Answer from the drawing. Dimensions are ordinates in mm from the lowest x, y and z of the part. A direction names the side the tool comes from. Round coordinates to 2 decimals unless told otherwise and drop trailing zeros. Write each loop counter-clockwise with the first axis right and the second up, starting at its lowest first coordinate (ties: lowest second). Pieces come first, ordered by that corner, then holes. Notation, with made-up numbers: (-9, 43.5) - (48, 43.5) arc R10 ccw to (48, 61.5) - close; hole circle Ø3 at (35, 13). An arc over 180 degrees is marked (long way). Answer in a Markdown table with one row per item.
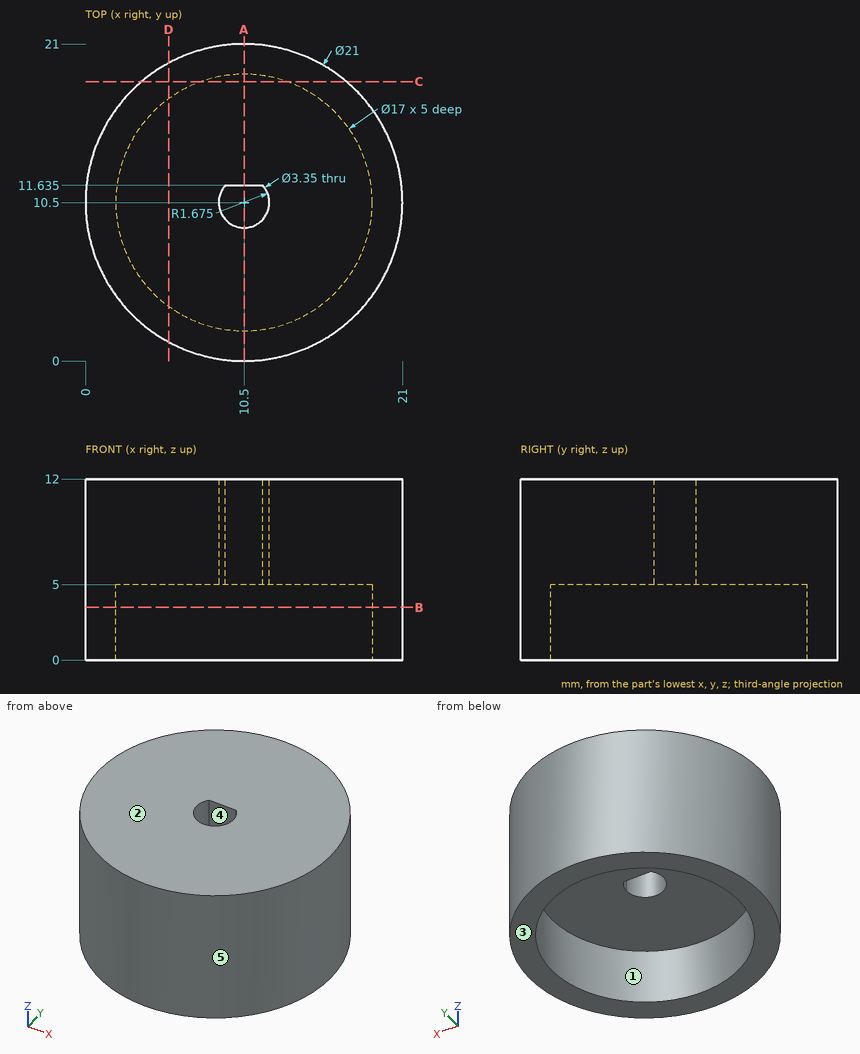
(1) Section B-B (z = 3.5) is taken. Give the vertices of the cut face in (x, y), and give its area (3 significant figures).
Checked values:
| item | result |
|---|---|
| outline | circle Ø21 at (10.5, 10.5); hole circle Ø17 at (10.5, 10.5) |
| area | 119 mm2 |
(2) Section A-A (x = 10.5) is taken. Give the vertices of the cut face in (y, z) (1 decimal), and give its area (3 significant figures).
Checked values:
| item | result |
|---|---|
| outline | (0, 0) - (2, 0) - (2, 5) - (8.8, 5) - (8.8, 12) - (0, 12) - close; (11.6, 5) - (19, 5) - (19, 0) - (21, 0) - (21, 12) - (11.6, 12) - close |
| area | 147 mm2 |
(3) For a pull along X with two mould halves and no side action, classify the marked faces 3, 4 and 5 as pulls with the +X half, pulls with the -X half, needs draft (parallel to the pull), parting line crosses it, or undercut.
Checked values:
| item | result |
|---|---|
| face 3 | needs draft |
| face 4 | undercut |
| face 5 | parting line crosses it |
(4) Section D-D (x = 5.5) is taken. Give the vertices of the cut face in (y, z).
Checked values:
| item | result |
|---|---|
| outline | (1.27, 0) - (3.63, 0) - (3.63, 5) - (17.37, 5) - (17.37, 0) - (19.73, 0) - (19.73, 12) - (1.27, 12) - close |
(5) For the marked faces 1 and 2, determine the directions among +Z, -Z, +X, -X, +Y, -Y from which every point of the face is accessible in a straight line to the end or side of a thin tool.
Checked values:
| item | result |
|---|---|
| face 1 | -Z |
| face 2 | +Z, +X, -X, +Y, -Y |
(6) Flat-ended cylindrical pins translate along their axes: pin 1 (10 mm diameter, centred on x = 10.5, y = 10.5, fed in from -Z); pin 2 (1.5 mm diameter, centred on y = 11.5, z = 7, fed in from +X); pin 3 (1.5 mm diameter, centred on x = 16.5, z = 4.5, fed in from +Y). Find the tip coordinate at first contact, or state that the pin passes through.
Checked values:
| item | result |
|---|---|
| pin 1 | stops at z = 5 |
| pin 2 | stops at x = 21 |
| pin 3 | stops at y = 19.59 |
(7) Section C-C (y = 18.5) is taken. Give the vertices of the cut face in (x, z).
Checked values:
| item | result |
|---|---|
| outline | (3.7, 0) - (7.63, 0) - (7.63, 5) - (13.37, 5) - (13.37, 0) - (17.3, 0) - (17.3, 12) - (3.7, 12) - close |
(8) Find the intervals of material crossed by line 1 (Y direction, x = 10.5, z = 1.4); line 2 (Z direction, x = 11, y = 11.75); line 3 (Y direction, x = 13.25, z = 1.5), in increasing order.
Checked values:
| item | result |
|---|---|
| line 1 | y = 0 to 2, 19 to 21 |
| line 2 | z = 5 to 12 |
| line 3 | y = 0.37 to 2.46, 18.54 to 20.63 |
